Geometry: final body of the model. Coordinates: model frame, mm. Face numbers are marked on the shaded views. Coordinates: 2 decimals unless noted, no trailing zeros. Loops run counter-clockwise (first coordinate to the right, second up) from the corner with the lowest first, then second, coordinate; pieces in that order, holes last. Notation, with made-up numbers: (-20, -26.75) - (2, -26.75) arc R31 ccw to (2, -1.75) - close; hole circle Ø7 at (-3.5, 26). An arc over 180 degrees is marked (long way). Answer in a Markdown table with one row per item.
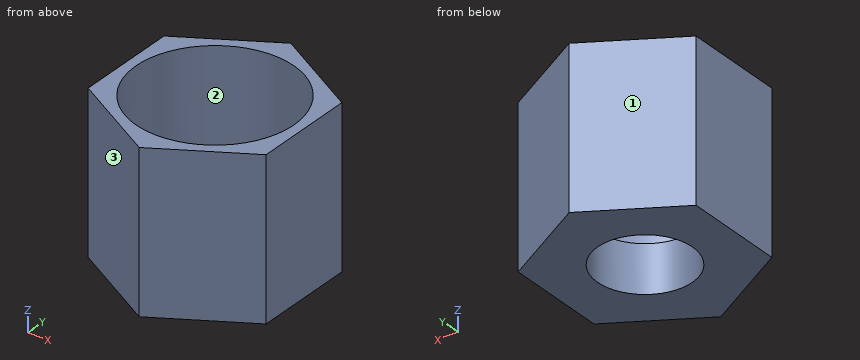
Autodesk Inventor part; units mm, degrees
ref_plane "YZ Plane" through (0, 0, 0) normal (1, 0, 0) x (0, 1, 0)
ref_plane "XZ Plane" through (0, 0, 0) normal (0, 1, 0) x (-1, 0, 0)
ref_plane "XY Plane" through (0, 0, 0) normal (0, 0, 1) x (1, 0, 0)
sketch "Sketch1" plane through (0, 0, 0) normal (0, 0, 1) x (1, 0, 0)
  line L0 (0, 6.5) -> (5.6292, 3.25)
  line L1 (5.6292, 3.25) -> (5.6292, -3.25)
  line L2 (5.6292, -3.25) -> (0, -6.5)
  line L3 (0, -6.5) -> (-5.6292, -3.25)
  line L4 (-5.6292, -3.25) -> (-5.6292, 3.25)
  line L5 (-5.6292, 3.25) -> (0, 6.5)
  point P0 (0, 0)
  point P1 (0, 0)
  dimension "d0" = 13
extrude "Extrusion1" add sketch "Sketch1" against normal blind 10
sketch "Sketch2" plane through (0, 0, 0) normal (0, 0, 1) x (1, 0, 0)
  point P0 (0, 0)
  point P1 (0, 0)
hole "Hole1" at (0, 0, 0) direction (0, 0, -1) diameter 10 depth 7
thread "Thread1"
sketch "Sketch3" plane through (0, 0, -10) normal (0, 0, -1) x (-1, 0, 0)
  point P0 (0, 0)
  point P1 (0, 0)
hole "Hole2" at (0, 0, -10) direction (0, 0, 1) diameter 6 depth 4
properties part number "124"
(1) Ray query, probe 1 along X at (y, z) = (0, -7.8); probe 2 along Y at (x, z) = (1, -7.5); probe 3 along Y at (x, z) = (-1.5, -6). Return the intervals inside material, ascending.
Verdict:
| item | result |
|---|---|
| probe 1 | x = -5.63 to -3, 3 to 5.63 |
| probe 2 | y = -5.92 to -2.83, 2.83 to 5.92 |
| probe 3 | y = -5.63 to -4.77, 4.77 to 5.63 |
(2) Cut plane A-A on y = 0. Output: boundary loops of the cut face in (x, z), then the cut area to 3 significant figures.
Verdict:
| item | result |
|---|---|
| outline | (-5.63, -10) - (-3, -10) - (-3, -7) - (-5, -7) - (-5, 0) - (-5.63, 0) - close; (3, -10) - (5.63, -10) - (5.63, 0) - (5, 0) - (5, -7) - (3, -7) - close |
| area | 24.6 mm² |
(3) Cut plane C-C on x = -1. Output: boundary loops of the cut face in (y, z).
Verdict:
| item | result |
|---|---|
| outline | (-5.92, -10) - (-2.83, -10) - (-2.83, -7) - (-4.9, -7) - (-4.9, 0) - (-5.92, 0) - close; (2.83, -10) - (5.92, -10) - (5.92, 0) - (4.9, 0) - (4.9, -7) - (2.83, -7) - close |
(4) Cut plane D-D on z = -9. Output: boundary loops of the cut face in (x, y), then the cut area to 3 significant figures.
Verdict:
| item | result |
|---|---|
| outline | (-5.63, -3.25) - (0, -6.5) - (5.63, -3.25) - (5.63, 3.25) - (0, 6.5) - (-5.63, 3.25) - close; hole circle Ø6 at (0, 0) |
| area | 81.5 mm² |
(5) Pull-direction query (Y, two-part tool) for the marked faces 1, 2 and 3; classes: pulls with the +Y half, pulls with the -Y half, needs draft (parallel to the pull), parting line crosses it, or undercut.
Verdict:
| item | result |
|---|---|
| face 1 | pulls with the +Y half |
| face 2 | undercut |
| face 3 | pulls with the -Y half |
(6) Cut plane B-B on z = -5.5. Output: boundary loops of the cut face in (x, y), then the cut area to 3 significant figures.
Verdict:
| item | result |
|---|---|
| outline | (-5.63, -3.25) - (0, -6.5) - (5.63, -3.25) - (5.63, 3.25) - (0, 6.5) - (-5.63, 3.25) - close; hole circle Ø10 at (0, 0) |
| area | 31.2 mm² |
(7) First-contact query: pin 1 Ø2 at (y, z) = (-3.5, -1.5) entering from -X; pin 2 Ø1 at (x, z) = (3, -7) entering from +Y; pin 3 Ø5 at (x, z) = (-3, -7) entering from +Y; pin 4 Ø5 at (x, y) = (-0.5, 0.5) entering from +Z. Flat tips, straight axial feed; report the tip coordinate or a pass-through.
Verdict:
| item | result |
|---|---|
| pin 1 | stops at x = -5.63 |
| pin 2 | stops at y = 5.06 |
| pin 3 | stops at y = 6.21 |
| pin 4 | stops at z = -7 |
